from build123d import *

# Parameters (mm, degrees)
CUT_EXTRUDE1_DEPTH      = 19.75
CUT_EXTRUDE1_DEPTH_BACK = 19.75


with BuildPart() as part:
    # Sketch1 → Revolve1 (revolve)
    with BuildSketch(Plane(origin=(0, 0, 0), x_dir=(0, 0, -1), z_dir=(1, 0, 0))):
        with BuildLine():
            ThreePointArc((18.75, -80), (13.258252147, -93.258252147), (0, -98.75))
            Line((0, -98.75), (0, -80))
            Line((0, -80), (11.25, -80))
            Line((11.25, -80), (11.25, 0))
            Line((11.25, 0), (18.75, 0))
            Line((18.75, 0), (18.75, -80))
        make_face()
    revolve(axis=Axis((0, -1981.522753143, 0), (0, 1, 0)))

    # Sketch1<3> → Cut-Extrude1 (cut, two sides)
    with BuildSketch(Plane(origin=(0, 0, 0), x_dir=(0, 0, -1), z_dir=(1, 0, 0))) as cut_extrude1_sk:
        with BuildLine():
            Line((-2.05, -16), (-2.05, -41))
            ThreePointArc((-2.05, -41), (0, -43.05), (2.05, -41))
            Line((2.05, -41), (2.05, -16))
            ThreePointArc((2.05, -16), (0, -13.95), (-2.05, -16))
        make_face()
    extrude(amount=CUT_EXTRUDE1_DEPTH, mode=Mode.SUBTRACT)
    extrude(cut_extrude1_sk.sketch, amount=-CUT_EXTRUDE1_DEPTH_BACK, mode=Mode.SUBTRACT)


solid = part.part
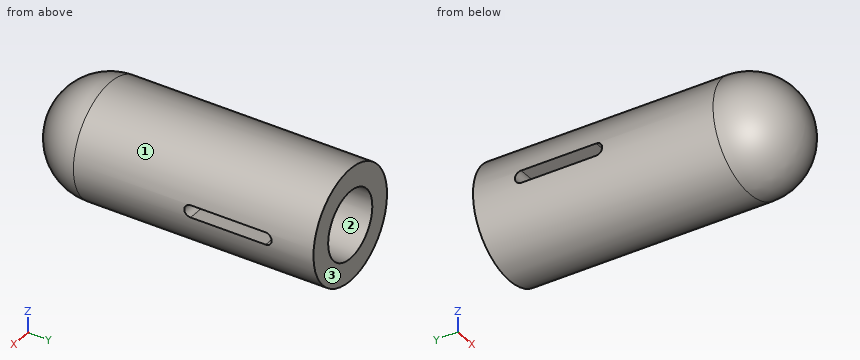
The model under review builds one solid part; all positions refer to its coordinate system, in mm. Face numbers are marked on the shaded views. Give positions to 0.01 mm unless a question says otherwise; leave off trailing zeros. Loops run counter-clockwise (first coordinate to the right, second up) from the corner with the lowest first, then second, coordinate; pieces in that order, holes last. Notation, with made-up numbers: (-16, 5) -> (15, 5) arc R22 cw to (15, 37) -> close; hole circle Ø7 at (29.25, 43.25). An arc over 180 degrees is marked (long way). Put each result on its own line as item: value. Start each with the question number.
1. Mouldability with a two-part tool opening along X and no side actions: class the marked faces 1, 2 and 3 as released by +X, released by -X, zero draft, split by the parting line, or undercut.
2. We need section D-D on z = -15. State the section outline as (x, y) points, then the cut area to 3 significant figures.
3. We need section C-C on x = 16.5. State the section outline as (y, z) points.
4. We need section A-A on z = 0. State the section outline as (x, y) points.
5. Clearance check with flat-ended pins moving along their axes: P1, Ø5, axis at y = -61.5, z = -10, coming from the +X side; P2, Ø2.5, axis at x = -13.5, y = -32, coming from the -Z side; P3, Ø8, axis at x = -4.5, z = 0.5, coming from the +Y side. State where each tip first meets the part, or that it passes through.
6. We need section B-B on x = 0. State the section outline as (y, z) points.
7. Wall thickness on probe 1 along Z at (x, y) = (2, -13); probe 2 along Z at (x, y) = (0, -50.5); probe 3 along X at (y, z) = (-45, 1.5): over which ranges is each line inside the solid? List them lowest first.
Determined:
1. face 1: split by the parting line
1. face 2: undercut
1. face 3: zero draft
2. outline: (-11.25, -80) arc R11.25 ccw to (11.25, -80) -> (11.25, 0) -> (-11.25, 0) -> close
2. area: 2,000 mm^2
3. outline: (-80, -8.91) -> (0, -8.91) -> (0, 8.91) -> (-80, 8.91) arc R8.91 ccw to start; hole (-41, -2.05) -> (-16, -2.05) arc R2.05 ccw to (-16, 2.05) -> (-41, 2.05) arc R2.05 ccw to start
4. outline: (-18.75, -80) arc R18.75 ccw to (18.75, -80) -> (18.75, -43.05) -> (11.25, -43.05) -> (11.25, -80) -> (-11.25, -80) -> (-11.25, -43.05) -> (-18.75, -43.05) -> close; (-18.75, -13.95) -> (-11.25, -13.95) -> (-11.25, 0) -> (-18.75, 0) -> close; (11.25, -13.95) -> (18.75, -13.95) -> (18.75, 0) -> (11.25, 0) -> close
5. P1: x = 17.18
5. P2: z = -14.2
5. P3: y = -80
6. outline: (-80, -18.75) -> (0, -18.75) -> (0, -11.25) -> (-80, -11.25) -> (-80, 11.25) -> (0, 11.25) -> (0, 18.75) -> (-80, 18.75) arc R18.75 ccw to start
7. probe 1: -18.64 to -11.07, 11.07 to 18.64
7. probe 2: -18.75 to -11.25, 11.25 to 18.75
7. probe 3: -18.69 to -11.15, 11.15 to 18.69
